Autodesk Inventor part; units mm, degrees
ref_plane "YZ Plane" through (0, 0, 0) normal (1, 0, 0) x (0, 1, 0)
ref_plane "XZ Plane" through (0, 0, 0) normal (0, 1, 0) x (-1, 0, 0)
ref_plane "XY Plane" through (0, 0, 0) normal (0, 0, 1) x (1, 0, 0)
sketch "スケッチ1" plane through (0, 0, 0) normal (0, 1, 0) x (-1, 0, 0)
  circle A0 centre (0, 0) radius 21
  dimension "d0" = 42
extrude "押し出し1" add sketch "スケッチ1" along normal blind 47
sketch "スケッチ2" plane through (0, 47, 0) normal (0, 1, 0) x (1, 0, 0)
  line L0 (0, 0) -> (0, 11.5)
  line L1 (0, 11.5) -> (0, -11.5)
  line L2 (-4.899, -11.5) -> (4.899, -11.5)
  line L3 (-4.899, 11.5) -> (4.899, 11.5)
  arc A0 (-4.899, 11.5) -> (-4.899, -11.5) centre (0, 0) ccw
  arc A1 (4.899, -11.5) -> (4.899, 11.5) centre (0, 0) ccw
extrude "押し出し2" add sketch "スケッチ2" along normal blind 2
sketch "スケッチ3" plane through (0, 47, 0) normal (0, 1, 0) x (1, 0, 0)
  circle A0 centre (0, 0) radius 17.5
  point P0 (-17.5, 0)
  point P1 (0, 17.5)
  point P2 (0, -17.5)
  point P3 (17.5, 0)
  dimension "d8" = 35
hole "穴1" at (-17.5, 47, 0) at (0, 47, -17.5) at (0, 47, 17.5) at (17.5, 47, 0) direction (0, -1, 0) diameter 4 end through all
sketch "スケッチ4" plane through (0, 49, 0) normal (0, 1, 0) x (1, 0, 0)
  circle A0 centre (0, 0) radius 4
  dimension "d16" = 8
extrude "押し出し3" add sketch "スケッチ4" along normal blind 20
sketch "スケッチ5" plane through (0, 0, 0) normal (0, -1, 0) x (1, 0, 0)
  circle A0 centre (0, 0) radius 23.25
  dimension "d19" = 46.5
extrude "押し出し4" add sketch "スケッチ5" along normal blind 59
properties part number "IG42-017"
Can you work these out from the model? Positions are in its coordinate system, mm. A direction names the side the tool comes from. Coordinates: 2 decimals unless noted, no trailing zeros. Write each loop counter-clockwise with the first axis right and the second up, starting at its lowest first coordinate (ties: lowest second). Pieces come first, ordered by that corner, then holes. Notation, with made-up numbers: (-17.75, 54) - (6.25, 54) arc R17 cw to (6.25, 60) - close; hole circle Ø9 at (18.25, -39.75). An arc over 180 degrees is marked (long way). Return JSON: item names as keys, results as strings.
Q1. If we section it at B-B (z = 0): Please give me the cut outline in (x, y).
Computed values:
{"outline": "(-23.25, -59) - (23.25, -59) - (23.25, 0) - (21, 0) - (21, 47) - (19.5, 47) - (19.5, 0) - (15.5, 0) - (15.5, 47) - (12.5, 47) - (12.5, 49) - (4, 49) - (4, 69) - (-4, 69) - (-4, 49) - (-12.5, 49) - (-12.5, 47) - (-15.5, 47) - (-15.5, 0) - (-19.5, 0) - (-19.5, 47) - (-21, 47) - (-21, 0) - (-23.25, 0) - close"}
Q2. On a 3-axis mill with a long thin cutter (end or side, diameter ignored), from which of +Z, -Z, +X, -X, +Y, -Y can I reach the whole of each face in a straight line? I mean faces 5 (the cylindrical face through (-12.5, 48, 0.2)), 6 (the flat face through (0, -59, 0)), 7 (the flat face through (-5, 0, -21)). Say none if no direction works.
Computed values:
{"face 5": "-X, +Y", "face 6": "+Z, -Z, +X, -X, -Y", "face 7": "+Y"}
Q3. Please list where these lines run through material, in increasing order: L1, parallel to Z at x = 0, y = 26; L2, parallel to Y at x = 1.5, z = -20.5; L3, parallel to Y at x = 1, z = -16. Write a range as from..to.
Computed values:
{"L1": "z = -21..-19.5, -15.5..15.5, 19.5..21", "L2": "y = -59..47", "L3": "y = -59..0"}
Q4. If we section it at C-C (y = -8): Please give me the cut outline in (x, z), then the cut area to 3 significant figures.
Computed values:
{"outline": "circle Ø46.5 at (0, 0)", "area": "1,700 mm2"}
Q5. If we section it at A-A (x = 0): Please give me the cut outline in (y, z), then the cut area to 3 significant figures.
Computed values:
{"outline": "(-59, -23.25) - (0, -23.25) - (0, -21) - (47, -21) - (47, -19.5) - (0, -19.5) - (0, -15.5) - (47, -15.5) - (47, -11.5) - (49, -11.5) - (49, -4) - (69, -4) - (69, 4) - (49, 4) - (49, 11.5) - (47, 11.5) - (47, 15.5) - (0, 15.5) - (0, 19.5) - (47, 19.5) - (47, 21) - (0, 21) - (0, 23.25) - (-59, 23.25) - close", "area": "4,550 mm2"}
Q6. I'm going to push flat-ended pins straight in: pin 1 Ø2 at (x, z) = (18.5, 6.5) entering from +Y; pin 2 Ø3 at (y, z) = (35, 17) entering from -X; pin 3 Ø10 at (x, y) = (-17.5, 17.5) entering from -Z. Where does each tip first touch, or does it pass through?
Computed values:
{"pin 1": "stops at y = 47", "pin 2": "stops at x = -14.17", "pin 3": "stops at z = -16.87"}
Q7. Thinking about a two-plate mould opening in X: for faces 1 (the cylindrical face through (-20.03, 23.17, -6.31)), 2 (the flat face through (17, 0, 0)), 3 (the cylindrical face through (12.5, 48, -0.2)), 4 (the flat face through (-9, 47, -9)), which applies, +X half, -X half, draft (parallel to the pull), parting line (faces both ways), or undercut?
Computed values:
{"face 1": "parting line", "face 2": "undercut", "face 3": "+X half", "face 4": "draft"}
Q8. If we section it at D-D (z = 17): Please give me the cut outline in (x, y).
Computed values:
{"outline": "(-15.86, -59) - (15.86, -59) - (15.86, 0) - (12.33, 0) - (12.33, 47) - (1.94, 47) - (1.94, 0) - (-1.94, 0) - (-1.94, 47) - (-12.33, 47) - (-12.33, 0) - (-15.86, 0) - close"}
